Read the model definition and answer for the solid it produces. Units are mm, in the model's axes. Coordinates: 2 decimals unless noted, no trailing zeros. Write each loop counter-clockwise with the first axis right and the second up, starting at its lowest first coordinate (ties: lowest second). Pieces come first, ordered by that corner, then holes.
from build123d import *

# Parameters (mm, degrees)
ESQUISSE1_W                  = 18
ESQUISSE1_H                  = 154
ENL_V_MAT_EXTRU_1_REACH      = 160.117
ENL_V_MAT_EXTRU_1_END_RADIUS = 18
CHANFREIN1_SIZE              = 1
CHANFREIN2_SIZE              = 1


with BuildPart() as part:
    # Esquisse1 → Révolution1 (revolve)
    with BuildSketch(Plane.XY, mode=Mode.PRIVATE) as r_volution1_sk:
        with Locations((9, 77)):
            Rectangle(ESQUISSE1_W, ESQUISSE1_H)
    revolve(r_volution1_sk.sketch.rotate(Axis((0, 154, 0), (0, -1, 0)), 270), axis=Axis((0, 154, 0), (0, -1, 0)))

    # Enlèv. mat.-Extru.1: up to this cylinder (the profile starts inside it)
    enl_v_mat_extru_1_end = Plane(origin=(0, 63.5, 0), z_dir=(0, -1, 0)) * Cylinder(ENL_V_MAT_EXTRU_1_END_RADIUS, 357.234, mode=Mode.PRIVATE)
    # Esquisse2 → Enlèv. mat.-Extru.1 (cut, up to the surface)
    with BuildSketch(Plane(origin=(0, 0, 13), x_dir=(-1, 0, 0), z_dir=(0, 0, -1)), mode=Mode.PRIVATE) as enl_v_mat_extru_1_sk1:
        with BuildLine():
            Line((-4.5, 94), (-4.5, 33))
            ThreePointArc((-4.5, 33), (0, 28.5), (4.5, 33))
            Line((4.5, 33), (4.5, 94))
            ThreePointArc((4.5, 94), (0, 98.5), (-4.5, 94))
        make_face()
    enl_v_mat_extru_1_tool1 = extrude(enl_v_mat_extru_1_sk1.sketch, amount=-ENL_V_MAT_EXTRU_1_REACH, mode=Mode.PRIVATE) & enl_v_mat_extru_1_end
    add(enl_v_mat_extru_1_tool1.solids().sort_by_distance((0, 63.5, 13))[0], mode=Mode.SUBTRACT)

    # Chanfrein1
    chanfrein1_edges = [part.edges().sort_by_distance(p)[0] for p in [
        (0, 154, 18),
    ]]
    chamfer(chanfrein1_edges, length=CHANFREIN1_SIZE)

    # Chanfrein2
    chanfrein2_edges = [part.edges().sort_by_distance(p)[0] for p in [
        (0, 0, 18),
    ]]
    chamfer(chanfrein2_edges, length=CHANFREIN2_SIZE)


solid = part.part
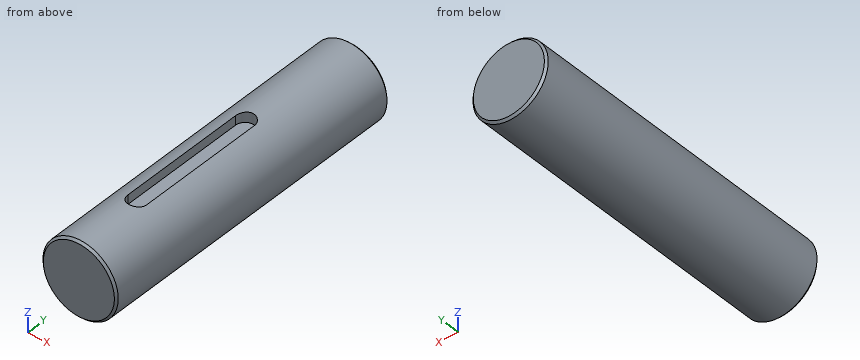
Item 1: The part is cut by section A-A (x = 0). Give the vertices of the cut face in (y, z).
Item 2: Find the intervals of material crossed by probe 1 along Z at (x, y) = (-0.5, 53.5); probe 2 along Z at (x, y) = (11, 71); probe 3 along X at (y, z) = (74, 12), in increasing order.
Item 3: The part is cut by section B-B (y = 53). Give the vertices of the cut face in (x, z), and give its area (3 significant figures).
Item 4: Given pin 1 (3 mm diameter, centred on x = -14.5, y = 24, fed in from +Z); pin 2 (5 mm diameter, centred on y = 56.5, z = 14, fed in from -X); pin 3 (5 mm diameter, centred on y = 53, z = 15, fed in from +X), each flat-ended and moving along its own axis, determine where each tip first touches the part or whether it passes through.
Item 5: The part is cut by section C-C (y = 18.5). Give the vertices of the cut face in (x, z), and give its area (3 significant figures).
Answer:
1. outline: (0, -17) - (1, -18) - (153, -18) - (154, -17) - (154, 17) - (153, 18) - (98.5, 18) - (98.5, 13) - (28.5, 13) - (28.5, 18) - (1, 18) - (0, 17) - close
2. probe 1: z = -17.99 to 13
2. probe 2: z = -14.25 to 14.25
2. probe 3: x = -13.42 to 13.42
3. outline: (-4.5, 13) - (-4.5, 17.43) arc R18 ccw (long way) to (4.5, 17.43) - (4.5, 13) - close
3. area: 975 mm2
4. pin 1: stops at z = 12.45
4. pin 2: stops at x = -13.85
4. pin 3: stops at x = 12.95
5. outline: circle Ø36 at (0, 0)
5. area: 1,020 mm2
